Study the drawing (mm; zero at the part's minimum x, y, z) and answer. Round coordinates to 2 decimals unless told otherwise and drop trailing zeros. Write each loop counter-clockwise with the first axis right and the second up, starting at its lowest first coordinate (ties: lowest second). Pieces come first, ordered by that corner, then holes. Notation, with made-up numbers: (52, -10.5) - (58, -10.5) arc R14 ccw to (58, 1.5) - close; hole circle Ø9 at (50, 74.5). An arc over 180 degrees is marked (long way). Return JSON: item names as keys, results as strings. Group by question number.
(1) Determine the mould class of the marked faces 1, 2 and 3 for opening direction Z: +Z half, -Z half, draft (parallel to the pull), parting line (faces both ways), or undercut.
(2) Section A-A, the plane y = 14 is taken. Give the number of separate pieces and of enclosed holes in the cut face, then the cut area to 3 significant figures.
(3) Section B-B, the plane z = 21.5 is taken. Write down the section's boundary in (x, y).
(4) This flat-tipped pin is pushed along its axis until it touches: pin 1 (7 mm diameter, centred on y = 9, z = 15.5, fed in from -X). Where does it stop, or does it pass through?
(5) Section D-D, the plane z = 17.5 is taken. Write down the section's boundary in (x, y), then the cut area to 3 significant figures.
(6) Section C-C, the plane x = 64 is taken. Write down the section's boundary in (y, z) (1 decimal), then the cut area to 3 significant figures.
(7) Find the intervals of material crossed by line 1 along Y through (x, z) = (8.89, 3.25); line 2 along Z through (x, y) = (59.69, 7); line 3 along Z through (x, y) = (63, 3.75) (1 decimal), in increasing order. Write a range as [from, to].
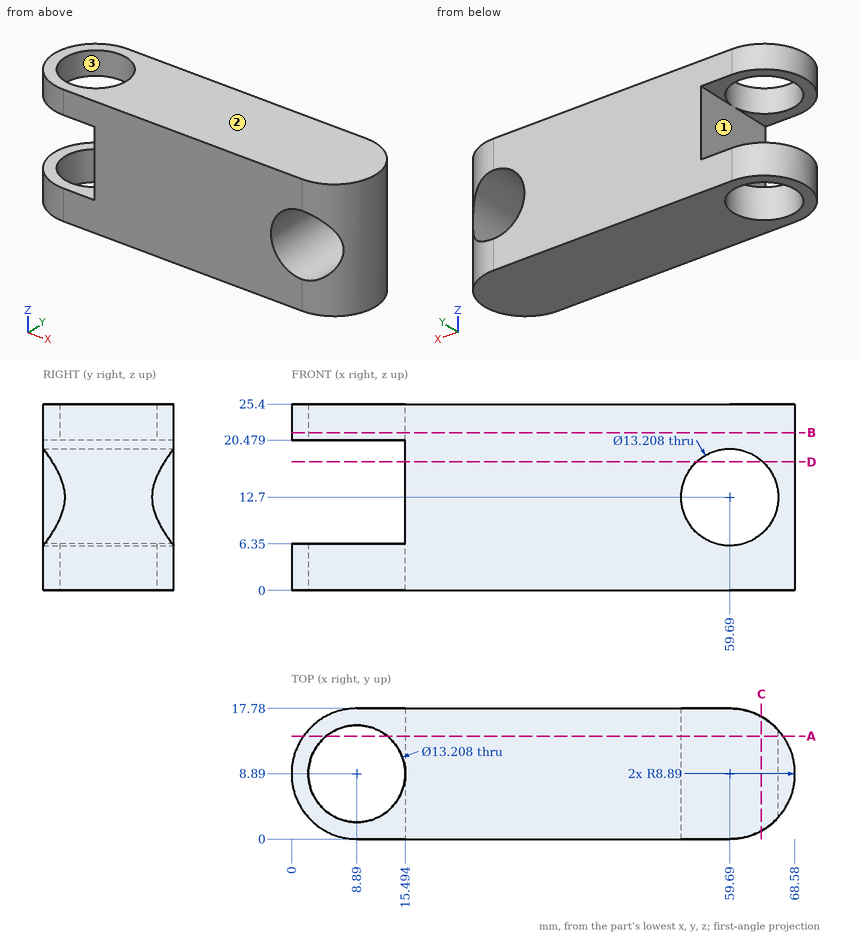
Working result:
{
 "1": {"face 1": "undercut", "face 2": "+Z half", "face 3": "draft"},
 "2": {"separate pieces": "3", "enclosed holes": "1", "area": "1,230 mm^2"},
 "3": {"outline": "(8.89, 0) - (59.69, 0) arc R8.89 ccw to (59.69, 17.78) - (8.89, 17.78) arc R8.89 ccw to start; hole circle Ø13.21 at (8.89, 8.89)"},
 "4": {"pin 1": "stops at x = 15.49"},
 "5": {"outline": "(15.49, 0) - (55.15, 0) - (55.15, 17.78) - (15.49, 17.78) - close; (64.23, 1.24) arc R8.89 ccw to (64.23, 16.54) - close", "area": "752 mm^2"},
 "6": {"outline": "(1.1, 0) - (16.7, 0) - (16.7, 7.7) - (1.1, 7.7) - close; (1.1, 17.7) - (16.7, 17.7) - (16.7, 25.4) - (1.1, 25.4) - close", "area": "239 mm^2"},
 "7": {"line 1": "y = [0, 2.29], [15.49, 17.78]", "line 2": "z = [0, 6.1], [19.3, 25.4]", "line 3": "z = [0, 7], [18.4, 25.4]"}
}
